Can you work these out from the model? Positions are in its coordinate system, mm. Face numbers are marked on the shaded views. A direction names the side the tool comes from. Give positions to 0.01 mm unless a question says otherwise; leave off trailing zeros. Order: outer loops, then holes, each group sorted by start corner. A loop starts at its lowest first (then second) coordinate and runs counter-clockwise, first axis right, second up. Notation, with made-up numbers: (75.5, -32) - (92.5, -32) arc R19 ccw to (92.5, -2) - close; hole circle Ø5 at (14, -1.75). An arc over 180 degrees is marked (long way). Answer as a JSON object with one key per item and string values.
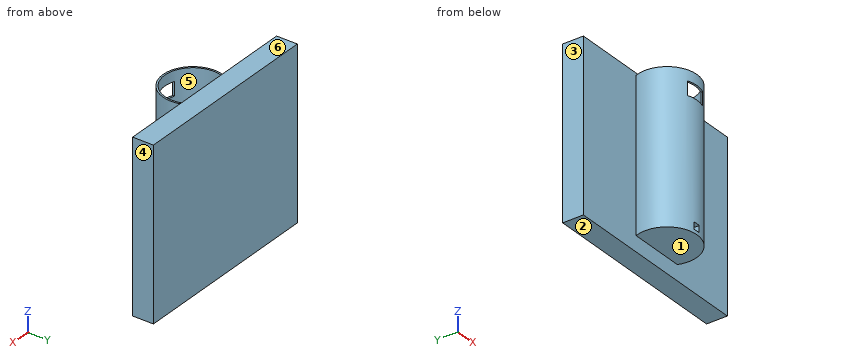
```python
from build123d import *

# Parameters (mm, degrees)
SKETCH_R             = 8.6
PAD_DEPTH            = 1
SKETCH001_R          = 8.6
SKETCH001_R_2        = 3.2
PAD001_DEPTH         = 6.6
SKETCH002_W          = 2
SKETCH002_H          = 2
POCKET_DEPTH         = 8.601
POCKET_DEPTH_BACK    = -8.601
SKETCH003_R          = 8.6
SKETCH003_R_2        = 8.1
PAD002_DEPTH         = 36
SKETCH004_W          = 6
SKETCH004_H          = 4
POCKET001_DEPTH      = 8.601
POCKET001_DEPTH_BACK = -8.601
SKETCH006_W          = 56.248293
SKETCH006_H          = 48.654014
PAD003_DEPTH         = 6


with BuildPart() as part:
    # Sketch → Pad (new body)
    with BuildSketch(Plane.XY):
        Circle(SKETCH_R)
    extrude(amount=PAD_DEPTH)

    # Sketch001 (on Face3 of Pad) → Pad001 (join)
    with BuildSketch(Plane.XY.offset(1)):
        Circle(SKETCH001_R)
        Circle(SKETCH001_R_2, mode=Mode.SUBTRACT)
    extrude(amount=PAD001_DEPTH)

    # Sketch002 → Pocket (cut, two sides)
    with BuildSketch(Plane.XZ) as pocket_sk:
        with Locations((0, 2)):
            Rectangle(SKETCH002_W, SKETCH002_H)
    extrude(amount=-POCKET_DEPTH, mode=Mode.SUBTRACT)
    extrude(pocket_sk.sketch, amount=-POCKET_DEPTH_BACK, mode=Mode.SUBTRACT)

    # Sketch003 (on Face12 of Pocket) → Pad002 (join)
    with BuildSketch(Plane.XY.offset(7.6)):
        Circle(SKETCH003_R)
        Circle(SKETCH003_R_2, mode=Mode.SUBTRACT)
    extrude(amount=PAD002_DEPTH)

    # Sketch004 → Pocket001 (cut, two sides)
    with BuildSketch(Plane.XZ) as pocket001_sk:
        with Locations((0, 38.6)):
            Rectangle(SKETCH004_W, SKETCH004_H)
    extrude(amount=-POCKET001_DEPTH, mode=Mode.SUBTRACT)
    extrude(pocket001_sk.sketch, amount=-POCKET001_DEPTH_BACK, mode=Mode.SUBTRACT)

    # Sketch006 (on DatumPlane) → Pad003 (join)
    with BuildSketch(Plane.XZ.offset(-9)):
        with Locations((-0.52784, 19.889832)):
            Rectangle(SKETCH006_W, SKETCH006_H)
    extrude(amount=PAD003_DEPTH)


solid = part.part
```
Q1. If we section it at D-D, the plane y = 0: Please give me the cut outline in (x, z).
Recorded:
{"outline": "(-8.6, 0) - (8.6, 0) - (8.6, 43.6) - (8.1, 43.6) - (8.1, 7.6) - (3.2, 7.6) - (3.2, 1) - (-3.2, 1) - (-3.2, 7.6) - (-8.1, 7.6) - (-8.1, 43.6) - (-8.6, 43.6) - close"}
Q2. If we section it at B-B, the plane y = -6.75: Please give me the cut outline in (x, z), then the cut area to 3 significant figures.
Recorded:
{"outline": "(-5.33, 0) - (5.33, 0) - (5.33, 43.6) - (4.48, 43.6) - (4.48, 7.6) - (-4.48, 7.6) - (-4.48, 43.6) - (-5.33, 43.6) - close; hole (-1, 1) - (1, 1) - (1, 3) - (-1, 3) - close", "area": "138 mm^2"}
Q3. I need wall thicknesses on L1, parallel to X at y = 0, z = 4.75; L2, parallel to X at y = 0, z = 21.5; L3, parallel to Y at x = 0, z = 22. Which ranges of each line are inside material? Lowest first, please.
Recorded:
{"L1": "x = -8.6 to -3.2, 3.2 to 8.6", "L2": "x = -8.6 to -8.1, 8.1 to 8.6", "L3": "y = -8.6 to -8.1, 3 to 9"}
Q4. If we section it at C-C, the plane z = 15: Please give me the cut outline in (x, y), then the cut area to 3 significant figures.
Recorded:
{"outline": "(-28.65, 3) - (-8.06, 3) arc R8.6 ccw (long way) to (8.06, 3) - (27.6, 3) - (27.6, 9) - (-28.65, 9) - close; hole (-7.52, 3) arc R8.1 ccw (long way) to (7.52, 3) - close", "area": "354 mm^2"}
Q5. If we section it at A-A, the plane x = 0: Please give me the cut outline in (y, z).
Recorded:
{"outline": "(-8.6, 0) - (3, 0) - (3, -4.44) - (9, -4.44) - (9, 44.22) - (3, 44.22) - (3, 1) - (-8.6, 1) - close; (-8.6, 3) - (-3.2, 3) - (-3.2, 7.6) - (-8.1, 7.6) - (-8.1, 36.6) - (-8.6, 36.6) - close; (-8.6, 40.6) - (-8.1, 40.6) - (-8.1, 43.6) - (-8.6, 43.6) - close"}
Q6. I'm going to push flat-ended pins straight in: pin 1 Ø1.5 at (x, y) = (-16.5, 1.5) entering from +Z; pin 2 Ø8 at (y, z) = (-4.5, 34) entering from +X; pin 3 Ø1.6 at (y, z) = (-7, 2.5) entering from -X; pin 4 Ø3.5 at (x, y) = (1.5, -5.5) entering from +Z. Where does each tip first touch, or does it pass through?
Recorded:
{"pin 1": "passes through", "pin 2": "stops at x = 8.59", "pin 3": "stops at x = -5.96", "pin 4": "stops at z = 7.6"}
Q7. Which directions (+Z, -Z, +X, -X, +Y, -Y) give clear straight access to the entire face, cutting with the end or side of a thin tool? Please do the marked faces 1 and 2.
Recorded:
{"face 1": "-Z, +X, -X, -Y", "face 2": "-Z, +X, -X, +Y, -Y"}
Q8. We'd pull the mould along X, two halves only. Please class the marked faces 3, 4, 5 and 6: released by +X, released by -X, zero draft, split by the parting line, or undercut.
Recorded:
{"face 3": "released by -X", "face 4": "released by +X", "face 5": "undercut", "face 6": "zero draft"}
